```python
from build123d import *

# Parameters (mm, degrees)
SKETCH28_W                                   = 80
SKETCH28_H                                   = 80
BOSS_EXTRUDE1_DEPTH                          = 10
CBORE_FOR_M10_CHEESE_HEAD_SCREW1_D           = 12
CBORE_FOR_M10_CHEESE_HEAD_SCREW1_CBORE_D     = 26
CBORE_FOR_M10_CHEESE_HEAD_SCREW1_CBORE_DEPTH = 5
SKETCH37_R                                   = 22.5
SKETCH37_R_2                                 = 15.5
CUT_EXTRUDE2_DEPTH                           = 6
CUT_EXTRUDE6_DEPTH                           = 6
SKETCH40_W                                   = 18.062589032
SKETCH40_H                                   = 3
BOSS_EXTRUDE7_DEPTH                          = 13
SKETCH47_W                                   = 10
SKETCH47_H                                   = 9.031294516
CUT_EXTRUDE12_DEPTH                          = 10
SKETCH41_R                                   = 33.75
SKETCH41_R_2                                 = 26.25
CUT_EXTRUDE7_DEPTH                           = 1.65
SKETCH36_R                                   = 1
CUT_EXTRUDE13_DEPTH                          = 10
SKETCH42_W                                   = 9.8
SKETCH42_H                                   = 11.037342061
CUT_EXTRUDE8_DEPTH                           = 2
CUT_EXTRUDE11_DEPTH                          = 20
SKETCH45_W                                   = 2.851047628
SKETCH45_H                                   = 9.955339391
BOSS_EXTRUDE8_DEPTH                          = 14
BOSS_EXTRUDE9_START                          = -9.955339
BOSS_EXTRUDE9_DEPTH                          = 9.955339


with BuildPart() as part:
    # Sketch28 → Boss-Extrude1 (new body)
    with BuildSketch(Plane(origin=(0, 0, 0), x_dir=(1, 0, 0), z_dir=(0, 1, 0))):
        with Locations((1.944585414, 4.241283073)):
            Rectangle(SKETCH28_W, SKETCH28_H)
    extrude(amount=BOSS_EXTRUDE1_DEPTH)

    # CBORE for M10 Cheese Head Screw1 (through all)
    with Locations(Plane(origin=(0, 10, 0), x_dir=(1, 0, 0), z_dir=(0, 1, 0))):
        with Locations((1.944585414, 4.241283073)):
            CounterBoreHole(CBORE_FOR_M10_CHEESE_HEAD_SCREW1_D / 2, CBORE_FOR_M10_CHEESE_HEAD_SCREW1_CBORE_D / 2, CBORE_FOR_M10_CHEESE_HEAD_SCREW1_CBORE_DEPTH)

    # Sketch37 → Cut-Extrude2 (cut)
    with BuildSketch(Plane(origin=(0, 10, 0), x_dir=(1, 0, 0), z_dir=(0, 1, 0))):
        with Locations(Location((1.944585414, 4.241283073, 0), (0, 0, 270))):
            Circle(SKETCH37_R)
        with Locations(Location((1.944585414, 4.241283073, 0), (0, 0, 270))):
            Circle(SKETCH37_R_2, mode=Mode.SUBTRACT)
    extrude(amount=-CUT_EXTRUDE2_DEPTH, mode=Mode.SUBTRACT)

    # Sketch39 → Cut-Extrude6 (cut)
    with BuildSketch(Plane(origin=(0, 10, 0), x_dir=(1, 0, 0), z_dir=(0, 1, 0))):
        with BuildLine():
            Line((6.944585414, -35.758716927), (6.944585414, -17.696127895))
            ThreePointArc((6.944585414, -17.696127895), (1.944585414, -18.258716927), (-3.055414586, -17.696127895))
            Line((-3.055414586, -17.696127895), (-3.055414586, -35.758716927))
            Line((-3.055414586, -35.758716927), (1.944585414, -35.758716927))
            Line((1.944585414, -35.758716927), (6.944585414, -35.758716927))
        make_face()
    extrude(amount=-CUT_EXTRUDE6_DEPTH, mode=Mode.SUBTRACT)

    # Sketch40 → Boss-Extrude7 (add)
    with BuildSketch(Plane(origin=(-3.055414586, 0, 0), x_dir=(0, 0, -1), z_dir=(1, 0, 0))):
        with Locations((-26.727422411, 8.5)):
            Rectangle(SKETCH40_W, SKETCH40_H)
    extrude(amount=BOSS_EXTRUDE7_DEPTH)

    # Sketch47 → Cut-Extrude12 (cut)
    with BuildSketch(Plane(origin=(0, 4, 0), x_dir=(1, 0, 0), z_dir=(0, 1, 0))):
        with Locations((1.944585414, -31.243069669)):
            Rectangle(SKETCH47_W, SKETCH47_H)
    extrude(amount=-CUT_EXTRUDE12_DEPTH, mode=Mode.SUBTRACT)

    # Sketch41 → Cut-Extrude7 (cut)
    with BuildSketch(Plane(origin=(0, 10, 0), x_dir=(1, 0, 0), z_dir=(0, 1, 0))):
        with Locations(Location((1.944585414, 4.241283073, 0), (0, 0, 270))):
            Circle(SKETCH41_R)
        with Locations(Location((1.944585414, 4.241283073, 0), (0, 0, 270))):
            Circle(SKETCH41_R_2, mode=Mode.SUBTRACT)
    extrude(amount=-CUT_EXTRUDE7_DEPTH, mode=Mode.SUBTRACT)

    # Sketch36 → Cut-Extrude13 (cut)
    with BuildSketch(Plane.XZ):
        with Locations(Location((12.444585414, -16.741283073, 0), (0, 0, 270))):
            Circle(SKETCH36_R)
        with Locations(Location((12.444585414, -4.241283073, 0), (0, 0, 270))):
            Circle(SKETCH36_R)
        with Locations(Location((-8.555414586, -16.741283073, 0), (0, 0, 16.545854879))):
            Circle(SKETCH36_R)
        with Locations(Location((-8.555414586, -4.241283073, 0), (0, 0, 270))):
            Circle(SKETCH36_R)
    extrude(amount=-CUT_EXTRUDE13_DEPTH, mode=Mode.SUBTRACT)

    # Sketch42 → Cut-Extrude8 (cut)
    with BuildSketch(Plane.XZ):
        with Locations((1.966640169, -13.109663986)):
            Rectangle(SKETCH42_W, SKETCH42_H)
    extrude(amount=-CUT_EXTRUDE8_DEPTH, mode=Mode.SUBTRACT)

    # Sketch43 → Cut-Extrude11 (cut)
    with BuildSketch(Plane(origin=(0, 10, 0), x_dir=(1, 0, 0), z_dir=(0, 1, 0))):
        with BuildLine():
            ThreePointArc((-38.055414586, 4.241282966), (-26.339685871, 32.525554283), (1.944585414, 44.241283073))
            Line((1.944585414, 44.241283073), (-38.055414586, 44.241283073))
            Line((-38.055414586, 44.241283073), (-38.055414586, 4.241282966))
        make_face()
        with BuildLine():
            ThreePointArc((1.944585414, -35.758716927), (-26.339685795, -24.042988212), (-38.055414586, 4.241282966))
            Line((-38.055414586, 4.241282966), (-38.055414586, -35.758716927))
            Line((-38.055414586, -35.758716927), (1.944585414, -35.758716927))
        make_face()
    extrude(amount=-CUT_EXTRUDE11_DEPTH, mode=Mode.SUBTRACT)

    # Sketch45 → Boss-Extrude8 (add)
    with BuildSketch(Plane(origin=(0, 8.35, 0), x_dir=(1, 0, 0), z_dir=(0, 1, 0))):
        with Locations((-32.810971356, 5.43037333)):
            Rectangle(SKETCH45_W, SKETCH45_H)
    extrude(amount=BOSS_EXTRUDE8_DEPTH)

    # Sketch46 → Boss-Extrude9 (add)
    with BuildSketch(Plane.XY.offset(-0.452703634).offset(BOSS_EXTRUDE9_START)):
        Polygon((-31.385447542, 22.35), (-31.385447542, 20.057188555), (-29.944471524, 20.057188555), align=None)
    extrude(amount=BOSS_EXTRUDE9_DEPTH)


solid = part.part
```
Geometry: final body of the model. Coordinates: model frame, mm. A direction names the side the tool comes from. Coordinates: 2 decimals unless noted, no trailing zeros. Loops run counter-clockwise (first coordinate to the right, second up) from the corner with the lowest first, then second, coordinate; pieces in that order, holes last. Notation, with made-up numbers: (-3.75, 77.25) -> (33.25, 77.25) arc R21 cw to (33.25, 90.25) -> close; hole circle Ø11 at (71, 2). An arc over 180 degrees is marked (long way). Use a Markdown table: item, result. Add a question column.
(1) Mould query, pull axis Z, two halves, no side actions, for faces 4 (the flat face through (2, 1, -18.628)), 5 (the flat face through (-33, 16, -10.408)), 6 (the flat face through (2, 7, 27)), 7 (the cylindrical face through (9.829, 9.187, 20.797)). Classes: pulls with the +Z half, pulls with the -Z half, needs draft (parallel to the pull), parting line crosses it, or undercut.
(2) Line query: line 1 along Z through (x, y) = (-10, 8); line 2 along X through (y, z) = (9.25, -10); line 3 along Y through (x, z) = (17, -25.5). Output: solid intervals per line, ascending.
(3) Section query A-A, the plane x = 1. State how many separate pieces and enclosed holes the cut face has, plus the area to 3 significant figures.
(4) Section query C-C, the plane x = 9. Return loops of the section in (y, z).
(5) Access query for faces 1 (the cylindrical face through (-0.87, 7.54, 8.45)), 2 (the flat face through (-3.055, 4, 28)), 3 (the flat face through (-2.933, 1, -13)). Directions: +Z, -Z, +X, -X, +Y, -Y. A direction counts if a zero-diameter tool reaches every point of the face in a straight line with its end or side. Return the directions, or none.
(6) Section query D-D, the plane y = 19. Return loops of the section in (x, z).
(7) Section query B-B, the plane z = 6. Return loops of the section in (x, y), plus the area to 3 significant figures.
(8) Pin query (flat end, axial travel): pin 1 Ø2.5 at (x, z) = (-8.56, -16.74) entering from +Y; pin 2 Ø1.6 at (x, z) = (-8.56, -4.24) entering from -Y; pin 3 Ø1.5 at (x, y) = (-2, 5.5) entering from +Z; pin 4 Ø2 at (x, y) = (-31.5, 15.5) entering from +Z. Return the tip coordinate at first contact, or that it passes through.
Answer:
| question | item | result |
|---|---|---|
| 1 | face 4 | undercut |
| 1 | face 5 | pulls with the -Z half |
| 1 | face 6 | needs draft |
| 1 | face 7 | undercut |
| 2 | line 1 | z = -42.42 to -23.31, -14.12 to -9.37, 0.89 to 5.64, 14.83 to 33.93 |
| 2 | line 2 | x = -37.64 to -31.31, -23.67 to -19.81, -12.45 to -9.71, 13.6 to 16.34, 23.7 to 27.56, 35.2 to 41.94 |
| 2 | line 3 | y = 0 to 10 |
| 3 | separate pieces | 3 |
| 3 | enclosed holes | 0 |
| 3 | area | 398 mm^2 |
| 4 | outline | (0, -44.24) -> (10, -44.24) -> (10, -37.25) -> (8.35, -37.25) -> (8.35, -29.53) -> (10, -29.53) -> (10, -25.61) -> (4, -25.61) -> (4, -18.04) -> (10, -18.04) -> (10, -15.16) -> (5, -15.16) -> (5, 6.68) -> (10, 6.68) -> (10, 9.56) -> (4, 9.56) -> (4, 17.12) -> (10, 17.12) -> (10, 21.04) -> (8.35, 21.04) -> (8.35, 28.76) -> (10, 28.76) -> (10, 35.76) -> (0, 35.76) -> close |
| 5 | face 1 | +Y |
| 5 | face 2 | +Z |
| 5 | face 3 | -Y |
| 6 | outline | (-34.24, -10.41) -> (-31.39, -10.41) -> (-31.39, -0.45) -> (-34.24, -0.45) -> close |
| 7 | outline | (-36.72, 0) -> (41.94, 0) -> (41.94, 10) -> (34.1, 10) -> (34.1, 8.35) -> (26.11, 8.35) -> (26.11, 10) -> (21.98, 10) -> (21.98, 4) -> (13.58, 4) -> (13.58, 10) -> (9.95, 10) -> (9.95, 5) -> (-6.06, 5) -> (-6.06, 10) -> (-9.69, 10) -> (-9.69, 4) -> (-18.09, 4) -> (-18.09, 10) -> (-22.23, 10) -> (-22.23, 8.35) -> (-30.21, 8.35) -> (-30.21, 10) -> (-36.72, 10) -> close |
| 7 | area | 579 mm^2 |
| 8 | pin 1 | stops at y = 10 |
| 8 | pin 2 | passes through |
| 8 | pin 3 | stops at z = 10.93 |
| 8 | pin 4 | stops at z = -0.45 |
